```python
from build123d import *

# Parameters (mm, degrees)
SKETCH3_W                        = 300
SKETCH3_H                        = 180
SKETCH3_R                        = 10
BOSS_EXTRUDE2_DEPTH              = 25
FILLET1_R                        = 10
FILLET2_R                        = 10
F_20_0MM_DOWEL_HOLE4_D           = 20
F_20_0MM_DOWEL_HOLE4_DEPTH       = 27.005
F_20_0MM_DOWEL_HOLE4_CSINK_D     = 20.05
F_20_0MM_DOWEL_HOLE4_CSINK_ANGLE = 45
F_20_0MM_DOWEL_HOLE4_TIP         = 6.00860619


with BuildPart() as part:
    # Sketch3 → Boss-Extrude2 (new body)
    with BuildSketch(Plane.XY):
        Rectangle(SKETCH3_W, SKETCH3_H)
        with Locations((-125, 65)):
            Circle(SKETCH3_R, mode=Mode.SUBTRACT)
        with Locations((-125, -65)):
            Circle(SKETCH3_R, mode=Mode.SUBTRACT)
        with Locations((0, 65)):
            Circle(SKETCH3_R, mode=Mode.SUBTRACT)
        with Locations((0, -65)):
            Circle(SKETCH3_R, mode=Mode.SUBTRACT)
        with Locations((125, 65)):
            Circle(SKETCH3_R, mode=Mode.SUBTRACT)
        with Locations((125, -65)):
            Circle(SKETCH3_R, mode=Mode.SUBTRACT)
    extrude(amount=BOSS_EXTRUDE2_DEPTH)

    # Fillet1
    fillet1_edges = [part.edges().sort_by_distance(p)[0] for p in [
        (-150, 90, 12.5),
    ]]
    fillet(fillet1_edges, radius=FILLET1_R)

    # Fillet2
    fillet2_edges = [part.edges().sort_by_distance(p)[0] for p in [
        (150, 90, 12.5),
        (150, -90, 12.5),
        (-150, -90, 12.5),
    ]]
    fillet(fillet2_edges, radius=FILLET2_R)

    # Sketch7 → Ø20.0mm Dowel Hole3 (revolve, cut)
    with BuildSketch(Plane(origin=(-125, 65, 25), x_dir=(0, -1, 0), z_dir=(1, 0, 0))):
        Polygon((0, 0), (0, 33.01360619), (10, 27.005), (10, 0.060355339), (10.025, 0), align=None)
    f_20_0mm_dowel_hole3 = revolve(axis=Axis((-125, 65, 31.35), (0, 0, -1)), mode=Mode.SUBTRACT)

    # Mirror2: Ø20.0mm Dowel Hole3 across plane
    add(f_20_0mm_dowel_hole3.mirror(Plane.XY.offset(25)), mode=Mode.SUBTRACT)

    # Ø20.0mm Dowel Hole4
    with Locations(Plane(origin=(-125, 65, 25), x_dir=(1, 0, 0), z_dir=(0, 0, 1))):
        with Locations((0, 0), (0, -130), (125, 0), (125, -130), (250, -130), (250, 0)):
            CounterSinkHole(F_20_0MM_DOWEL_HOLE4_D / 2, F_20_0MM_DOWEL_HOLE4_CSINK_D / 2, depth=F_20_0MM_DOWEL_HOLE4_DEPTH, counter_sink_angle=F_20_0MM_DOWEL_HOLE4_CSINK_ANGLE)
            with Locations((0, 0, -(F_20_0MM_DOWEL_HOLE4_DEPTH + F_20_0MM_DOWEL_HOLE4_TIP / 2))):  # 118° drill point
                Cone(0, F_20_0MM_DOWEL_HOLE4_D / 2, F_20_0MM_DOWEL_HOLE4_TIP, mode=Mode.SUBTRACT)


solid = part.part
```
Input: part model. Units: mm. Frame: model coordinates. Give positions to 0.01 mm unless a question says otherwise; leave off trailing zeros. Write each loop counter-clockwise with the first axis right and the second up, starting at its lowest first coordinate (ties: lowest second). Pieces come first, ordered by that corner, then holes. Notation, with made-up numbers: (72, 58) - (127, 58) arc R26 ccw to (127, 83) - close; hole circle Ø4 at (85.25, 85.5). An arc over 180 degrees is marked (long way). Write item = value, one per line. Start each with the question number.
1. Ray query, L1, parallel to X at y = 65, z = 10; L2, parallel to Y at x = 125, z = 6.5; L3, parallel to Y at x = 118.5, z = 22.5. Return the intervals inside material, ascending.
2. Mould query, pull axis X, two halves, no side actions, for faces 1 (the flat face through (-2, 1, 25)), 2 (the cylindrical face through (129.614, 56.128, 12.295)), 3 (the cylindrical face through (9.237, -68.83, 12.295)), 4 (the flat face through (150, -1, 12)). Classes: released by +X, released by -X, zero draft, split by the parting line, or undercut.
3. Section query A-A, the plane z = 11.5. Output: boundary loops of the cut face in (x, y).
4. First-contact query: pin 1 Ø12 at (x, y) = (-125, 65) entering from +Z. Flat tip, straight axial feed; report the tip coordinate or a pass-through.
5. Section query C-C, the plane y = 65. Output: boundary loops of the cut face in (x, z) (3 decimals), then the cut area to 3 significant figures.
6. Section query B-B, the plane x = -125. Output: boundary loops of the cut face in (y, z) (3 decimals).
Check sheet entries:
q1.L1 = -150 to -135, -115 to -10, 10 to 115, 135 to 150
q1.L2 = -90 to -75, -55 to 55, 75 to 90
q1.L3 = -90 to -72.6, -57.4 to 57.4, 72.6 to 90
q2.face_1 = zero draft
q2.face_2 = undercut
q2.face_3 = undercut
q2.face_4 = released by +X
q3.outline = (-150, -80) arc R10 ccw to (-140, -90) - (140, -90) arc R10 ccw to (150, -80) - (150, 80) arc R10 ccw to (140, 90) - (-140, 90) arc R10 ccw to (-150, 80) - close; hole circle Ø20 at (-125, -65); hole circle Ø20 at (-125, 65); hole circle Ø20 at (0, -65); hole circle Ø20 at (0, 65); hole circle Ø20 at (125, -65); hole circle Ø20 at (125, 65)
q4.pin_1 = through
q5.outline = (-150, 0) - (-135, 0) - (-135, 24.94) - (-135.025, 25) - (-150, 25) - close; (-115, 0) - (-10, 0) - (-10, 24.94) - (-10.025, 25) - (-114.975, 25) - (-115, 24.94) - close; (10, 0) - (115, 0) - (115, 24.94) - (114.975, 25) - (10.025, 25) - (10, 24.94) - close; (135, 0) - (150, 0) - (150, 25) - (135.025, 25) - (135, 24.94) - close
q5.area = 6,000 mm2
q6.outline = (-90, 0) - (-75, 0) - (-75, 24.94) - (-75.025, 25) - (-90, 25) - close; (-55, 0) - (55, 0) - (55, 24.94) - (54.975, 25) - (-54.975, 25) - (-55, 24.94) - close; (75, 0) - (90, 0) - (90, 25) - (75.025, 25) - (75, 24.94) - close
